```python
from build123d import *

# Parameters (mm, degrees)
BASE_FLANGE1_DEPTH          = 31.75
SKETCH6_R                   = 4.7625
CUT_EXTRUDE1_DEPTH          = 127
F_27_0_144_DIAMETER_HOLE1_D = 3.6576
SKETCH11_R                  = 6.35
CUT_EXTRUDE2_DEPTH          = 2.54


# Sheet-metal steps are written as plain solids
with BuildPart() as part:
    # Sketch1 → Base-Flange1 (new, symmetric)
    with BuildSketch(Plane.YZ):
        with BuildLine():
            Line((-31.75, -22.70125), (-31.75, 17.93875))
            ThreePointArc((-31.75, 17.93875), (-30.355096045, 21.306346045), (-26.9875, 22.70125))
            Line((-26.9875, 22.70125), (26.9875, 22.70125))
            ThreePointArc((26.9875, 22.70125), (30.355096045, 21.306346045), (31.75, 17.93875))
            Line((31.75, 17.93875), (31.75, -22.70125))
            Line((31.75, -22.70125), (30.1625, -22.70125))
            Line((30.1625, -22.70125), (30.1625, 17.93875))
            ThreePointArc((30.1625, 17.93875), (29.23256403, 20.18381403), (26.9875, 21.11375))
            Line((26.9875, 21.11375), (-26.9875, 21.11375))
            ThreePointArc((-26.9875, 21.11375), (-29.23256403, 20.18381403), (-30.1625, 17.93875))
            Line((-30.1625, 17.93875), (-30.1625, -22.70125))
            Line((-30.1625, -22.70125), (-31.75, -22.70125))
        make_face()
    extrude(amount=BASE_FLANGE1_DEPTH, both=True)

    # Sketch6 → Cut-Extrude1 (cut)
    with BuildSketch(Plane(origin=(0, 31.75, 0), x_dir=(-1, 0, 0), z_dir=(0, 1, 0))):
        with Locations(Location((0, 9.04875, 0), (0, 0, 270))):
            Circle(SKETCH6_R)
        with BuildLine():
            Line((-31.75, 9.04875), (-31.75, -117.95125))
            Line((-31.75, -117.95125), (31.75, -117.95125))
            Line((31.75, -117.95125), (31.75, 9.04875))
            ThreePointArc((31.75, 9.04875), (0, -22.70125), (-31.75, 9.04875))
        make_face()
    extrude(amount=-CUT_EXTRUDE1_DEPTH, mode=Mode.SUBTRACT)

    # #27 (0.144) Diameter Hole1 (through all)
    with Locations(Plane.XY.offset(22.70125)):
        with Locations((-25.4, 20.6375), (25.4, 20.6375), (25.4, -20.6375), (-25.4, -20.6375)):
            Hole(F_27_0_144_DIAMETER_HOLE1_D / 2)

    # Sketch11 → Cut-Extrude2 (cut)
    with BuildSketch(Plane.XY.offset(22.70125)):
        Circle(SKETCH11_R)
    extrude(amount=-CUT_EXTRUDE2_DEPTH, mode=Mode.SUBTRACT)


solid = part.part
```
Build history of the part. All positions in model axes, mm. A direction names the side the tool comes from. Round coordinates to 2 decimals unless told otherwise and drop trailing zeros. Write each loop counter-clockwise with the first axis right and the second up, starting at its lowest first coordinate (ties: lowest second). Pieces come first, ordered by that corner, then holes. Notation, with made-up numbers: (-12, -35) -> (-1, -35) arc R37 cw to (-1, 1) -> close; hole circle Ø3 at (40, 57). An arc over 180 degrees is marked (long way). Put each result on its own line as item: value.
Item 1: Slice it at A-A, the plane y = 0. Give the cut face in (x, z).
Here are the results:
outline: (-31.75, 21.11) -> (-6.35, 21.11) -> (-6.35, 22.7) -> (-31.75, 22.7) -> close; (6.35, 21.11) -> (31.75, 21.11) -> (31.75, 22.7) -> (6.35, 22.7) -> close
Item 2: Tool access for faces 4 (the face through (8, 0, 21.114)), 5 (the face through (-31.75, 0.1, 21.5)): list every direction of +Z, -Z, +X, -X, +Y, -Y with a clear straight run to the whole face (end or side of a thin tool).
Here are the results:
face 4: -Z, +X, -X
face 5: +Z, -Z, -X, +Y, -Y
Item 3: Flat gauge pins, fed straight in: P1, Ø3, axis at x = 25.4, y = 20.64, coming from the +Z side (1 decimal); P2, Ø6, axis at x = -25.4, y = 20.64, coming from the -Z side. Where does each tip first touch, or does it go through?
Here are the results:
P1: passes through
P2: stops at z = 21.11
Item 4: Two-plate mould, pull along X, no slides. Class faces 1 (the face through (-1.431, 30.967, 4.506)), 2 (the face through (0, -31.75, 2)), 3 (the face through (-0.698, 30.967, -22.694)): pulls with the +X half, pulls with the -X half, needs draft (parallel to the pull), parting line crosses it, or undercut.
Here are the results:
face 1: undercut
face 2: needs draft
face 3: parting line crosses it
Item 5: Slice it at C-C, the plane z = -19. Give the cut face in (x, y).
Here are the results:
outline: (-14.88, -31.75) -> (14.88, -31.75) -> (14.88, -30.16) -> (-14.88, -30.16) -> close; (-14.88, 30.16) -> (14.88, 30.16) -> (14.88, 31.75) -> (-14.88, 31.75) -> close
Item 6: Slice it at B-B, the plane x = 26. Count the separate pieces of the cut face and the enclosed holes in it, plus the area to 3 significant figures.
Here are the results:
separate pieces: 3
enclosed holes: 0
area: 181 mm^2
Item 7: Wall check: probe 1 along Y at (x, z) = (25.4, 21.5); probe 2 along Y at (x, z) = (25, 22) (3 decimals); probe 3 along Y at (x, z) = (19.5, 1). Give the ranges that are in metal, low to high. Write a range as from..to.
Here are the results:
probe 1: y = -30.15..-22.47, -18.81..18.81, 22.47..30.15
probe 2: y = -29.475..-22.422, -18.853..18.853, 22.422..29.475
probe 3: y = -31.75..-30.16, 30.16..31.75
